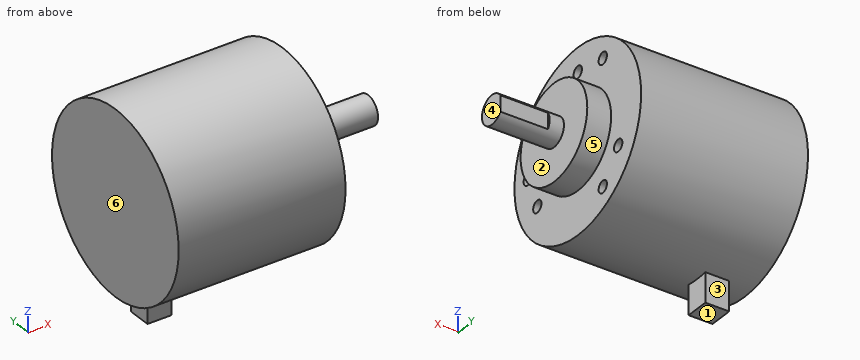
from build123d import *

# Parameters (mm, degrees)
SKETCH001_R  = 1.25
HOLE_DEPTH   = 7.248924
HOLE_TIPS_R  = 1.25
SKETCH002_W  = 20
SKETCH002_H  = 20
POCKET_DEPTH = 10
SKETCH003_W  = 5
SKETCH003_H  = 5
PAD_DEPTH    = 25


with BuildPart() as part:
    # Sketch → Revolution (revolve)
    with BuildSketch(Plane.XY):
        Polygon((0, 0), (0, 19), (35, 19), (35, 10), (40, 10), (40, 3), (53, 3), (53, 0), align=None)
    revolve(axis=Axis((0, 0, 0), (1, 0, 0)))

    # Sketch001 (on Face3 of Revolution) → Hole (cut)
    with BuildSketch(Plane.YZ.offset(35)):
        with Locations((-15, 0)):
            Circle(SKETCH001_R)
        with Locations((-12.124356, -7)):
            Circle(SKETCH001_R)
        with Locations((7.5, -12.990381)):
            Circle(SKETCH001_R)
        with Locations((12.124356, -7)):
            Circle(SKETCH001_R)
        with Locations((7.5, 12.990381)):
            Circle(SKETCH001_R)
        with Locations((0, 14)):
            Circle(SKETCH001_R)
    extrude(amount=-HOLE_DEPTH, mode=Mode.SUBTRACT)

    # Hole tips → Hole tip 1 section 0
    with BuildSketch(Plane.YZ.offset(27.751076), mode=Mode.PRIVATE) as hole_tip_1_s0:
        with Locations((-15, 0)):
            Circle(HOLE_TIPS_R)
    loft([hole_tip_1_s0.sketch, Vertex(27, -15, 0)], mode=Mode.SUBTRACT)

    # Hole tips → Hole tip 2 section 0
    with BuildSketch(Plane.YZ.offset(27.751076), mode=Mode.PRIVATE) as hole_tip_2_s0:
        with Locations((-12.124356, -7)):
            Circle(HOLE_TIPS_R)
    loft([hole_tip_2_s0.sketch, Vertex(27, -12.124356, -7)], mode=Mode.SUBTRACT)

    # Hole tips → Hole tip 3 section 0
    with BuildSketch(Plane.YZ.offset(27.751076), mode=Mode.PRIVATE) as hole_tip_3_s0:
        with Locations((7.5, -12.990381)):
            Circle(HOLE_TIPS_R)
    loft([hole_tip_3_s0.sketch, Vertex(27, 7.5, -12.990381)], mode=Mode.SUBTRACT)

    # Hole tips → Hole tip 4 section 0
    with BuildSketch(Plane.YZ.offset(27.751076), mode=Mode.PRIVATE) as hole_tip_4_s0:
        with Locations((12.124356, -7)):
            Circle(HOLE_TIPS_R)
    loft([hole_tip_4_s0.sketch, Vertex(27, 12.124356, -7)], mode=Mode.SUBTRACT)

    # Hole tips → Hole tip 5 section 0
    with BuildSketch(Plane.YZ.offset(27.751076), mode=Mode.PRIVATE) as hole_tip_5_s0:
        with Locations((7.5, 12.990381)):
            Circle(HOLE_TIPS_R)
    loft([hole_tip_5_s0.sketch, Vertex(27, 7.5, 12.990381)], mode=Mode.SUBTRACT)

    # Hole tips → Hole tip 6 section 0
    with BuildSketch(Plane.YZ.offset(27.751076), mode=Mode.PRIVATE) as hole_tip_6_s0:
        with Locations((0, 14)):
            Circle(HOLE_TIPS_R)
    loft([hole_tip_6_s0.sketch, Vertex(27, 0, 14)], mode=Mode.SUBTRACT)

    # Sketch002 (on Face19 of Hole) → Pocket (cut)
    with BuildSketch(Plane.YZ.offset(53)):
        with Locations((12.5, 0)):
            Rectangle(SKETCH002_W, SKETCH002_H)
    extrude(amount=-POCKET_DEPTH, mode=Mode.SUBTRACT)

    # Sketch003 → Pad (join)
    with BuildSketch(Plane.XY):
        with Locations((7.5, 0)):
            Rectangle(SKETCH003_W, SKETCH003_H)
    extrude(amount=-PAD_DEPTH)


solid = part.part
Work out the finished part from the listing and answer in its coordinate system (mm). Face numbers are marked on the shaded views. A direction names the side the tool comes from. Give positions to 0.01 mm unless a question says otherwise; leave off trailing zeros. Loops run counter-clockwise (first coordinate to the right, second up) from the corner with the lowest first, then second, coordinate; pieces in that order, holes last. Notation, with made-up numbers: (27, -36) -> (63, -36) arc R14 cw to (63, -16) -> close; hole circle Ø10 at (-25, 47). An arc over 180 degrees is marked (long way). Use a Markdown table: item, result. Add a question column.
1. Flat-ended cylindrical pins translate along their axes: pin 1 Ø8 at (x, z) = (47.5, -0.5) entering from +Y; pin 2 Ø3 at (y, z) = (7.5, -12.99) entering from +X; pin 3 Ø2 at (y, z) = (-12.12, -7) entering from +X. Find the tip coordinate at first contact, or state that the pin passes through.
2. Determine the mould class of the marked faces 4, 5 and 6 for opening direction X: released by +X, released by -X, zero draft, split by the parting line, or undercut.
3. Section C-C on z = -20 is taken. Determine the outline of the cut face in (x, y), and give its area (3 significant figures).
4. Section A-A on x = 32.5 is taken. Determine the outline of the cut face in (y, z), and give its area (3 significant figures).
5. For the marked faces 1, 2 and 3, determine the directions among +Z, -Z, +X, -X, +Y, -Y from which every point of the face is accessible in a straight line to the end or side of a thin tool.
6. Section B-B on y = -4 is taken. Determine the outline of the cut face in (x, z).
7. Find the intervals of material crossed by probe 1 along Z at (x, y) = (31.5, 0); probe 2 along Z at (x, y) = (32, 7); probe 3 along X at (y, z) = (-7, 17.5), in increasing order.
8. Section D-D on x = 48.5 is taken. Determine the outline of the cut face in (y, z).
Results below:
| question | item | result |
|---|---|---|
| 1 | pin 1 | stops at y = 2.5 |
| 1 | pin 2 | stops at x = 35 |
| 1 | pin 3 | stops at x = 27.6 |
| 2 | face 4 | released by +X |
| 2 | face 5 | zero draft |
| 2 | face 6 | released by -X |
| 3 | outline | (5, -2.5) -> (10, -2.5) -> (10, 2.5) -> (5, 2.5) -> close |
| 3 | area | 25.0 mm^2 |
| 4 | outline | circle Ø38 at (0, 0); hole circle Ø2.5 at (-15, 0); hole circle Ø2.5 at (-12.12, -7); hole circle Ø2.5 at (0, 14); hole circle Ø2.5 at (7.5, -12.99); hole circle Ø2.5 at (7.5, 12.99); hole circle Ø2.5 at (12.12, -7) |
| 4 | area | 1,100 mm^2 |
| 5 | face 1 | -Z, +X, -X, +Y, -Y |
| 5 | face 2 | +X |
| 5 | face 3 | -Z, +X, -X, +Y |
| 6 | outline | (0, -18.57) -> (35, -18.57) -> (35, -9.17) -> (40, -9.17) -> (40, 9.17) -> (35, 9.17) -> (35, 18.57) -> (0, 18.57) -> close |
| 7 | probe 1 | z = -19 to 12.75, 15.25 to 19 |
| 7 | probe 2 | z = -17.66 to -14.14, -11.84 to 11.84, 14.14 to 17.66 |
| 7 | probe 3 | x = 0 to 35 |
| 8 | outline | (2.5, -1.66) -> (2.5, 1.66) arc R3 ccw (long way) to start |
